from build123d import *

# Parameters (mm, degrees)
SKETCH1_W           = 155
SKETCH1_H           = 40
SKETCH1_R           = 9
BOSS_EXTRUDE1_DEPTH = 30
SKETCH2_W           = 155
SKETCH2_H           = 30
CUT_EXTRUDE1_DEPTH  = 21
SKETCH4_R           = 3.5
CUT_EXTRUDE3_DEPTH  = 31


with BuildPart() as part:
    # Sketch1 → Boss-Extrude1 (new body)
    with BuildSketch(Plane(origin=(0, 0, 0), x_dir=(1, 0, 0), z_dir=(0, 1, 0))):
        with Locations((7.5, 0)):
            Rectangle(SKETCH1_W, SKETCH1_H)
        Circle(SKETCH1_R, mode=Mode.SUBTRACT)
    extrude(amount=BOSS_EXTRUDE1_DEPTH)

    # Sketch2 → Cut-Extrude1 (cut, through all)
    with BuildSketch(Plane.XY):
        with Locations((7.5, 15)):
            Rectangle(SKETCH2_W, SKETCH2_H)
    extrude(amount=-CUT_EXTRUDE1_DEPTH, mode=Mode.SUBTRACT)

    # Sketch4 → Cut-Extrude3 (cut, through all)
    with BuildSketch(Plane.XZ):
        with Locations((-30, 9)):
            Circle(SKETCH4_R)
    extrude(amount=-CUT_EXTRUDE3_DEPTH, mode=Mode.SUBTRACT)


solid = part.part
Could you check a few things on this model? Use its own coordinates, in mm. Give positions to 0.01 mm unless a question says otherwise; leave off trailing zeros. Write each loop counter-clockwise with the first axis right and the second up, starting at its lowest first coordinate (ties: lowest second). Pieces come first, ordered by that corner, then holes. Notation, with made-up numbers: (-25.75, -30.5) -> (17.25, -30.5) arc R6 ccw to (17.25, -21.5) -> close; hole circle Ø4 at (46, -28). An arc over 180 degrees is marked (long way). Answer as a JSON object with one key per item and string values.
Q1. Please list where these lines run through material, in increasing order: L1, parallel to Z at x = -30, y = 10; L2, parallel to X at y = 13.5, z = 9.5; L3, parallel to X at y = 20.75, z = 11.25.
Taken from the geometry:
{"L1": "z = 0 to 5.5, 12.5 to 20", "L2": "x = -70 to -33.46, -26.54 to 85", "L3": "x = -70 to -32.68, -27.32 to 85"}
Q2. Suppose I cut it at C-C on z = 3.75. Write out the boundary of the cut face in (x, y), then the cut area to 3 significant figures.
Taken from the geometry:
{"outline": "(-70, 0) -> (-8.18, 0) -> (-8.18, 30) -> (-70, 30) -> close; (8.18, 0) -> (85, 0) -> (85, 30) -> (8.18, 30) -> close", "area": "4,160 mm²"}
Q3. Suppose I cut it at B-B on y = 6.75. Write out the boundary of the cut face in (x, z).
Taken from the geometry:
{"outline": "(-70, 0) -> (-9, 0) arc R9 cw to (9, 0) -> (85, 0) -> (85, 20) -> (-70, 20) -> close; hole circle Ø7 at (-30, 9)"}
Q4. We'd pull the mould along X, two halves only. Please class faces 1 (the flat face through (85, 15, 10)), 2 (the cylindrical face through (0, 15, 9)), 3 (the flat face through (6, 15, 20)): released by +X, released by -X, zero draft, split by the parting line, or undercut.
Taken from the geometry:
{"face 1": "released by +X", "face 2": "undercut", "face 3": "zero draft"}
Q5. Suppose I cut it at D-D on x = 0. Write out the boundary of the cut face in (y, z).
Taken from the geometry:
{"outline": "(0, 9) -> (30, 9) -> (30, 20) -> (0, 20) -> close"}
Q6. Suppose I cut it at A-A on x = -30. Write out the boundary of the cut face in (y, z).
Taken from the geometry:
{"outline": "(0, 0) -> (30, 0) -> (30, 5.5) -> (0, 5.5) -> close; (0, 12.5) -> (30, 12.5) -> (30, 20) -> (0, 20) -> close"}
